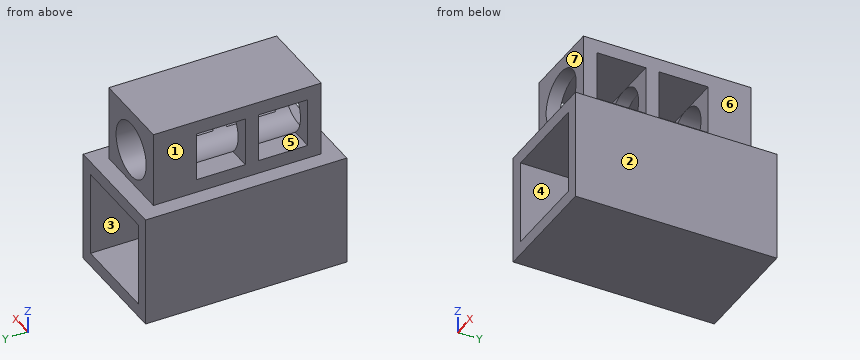
```python
from build123d import *

# Parameters (mm, degrees)
F0_W     = 13.2
F0_H     = 12.6
F1_DEPTH = 15
F0_W_2   = 12.3
F0_H_2   = 11.3
F0_R     = 4.15
F2_DEPTH = 12.5
F3_W     = 7.3
F3_H     = 7.3
F3_W_2   = 7.299999
F4_DEPTH = 25


with BuildPart() as f1:
    # F0 (on Front) → F1 (new body, symmetric)
    with BuildSketch(Plane.XZ):
        Polygon((8.6, -8.3), (8.6, 8.3), (6.15, 8.3), (-6.15, 8.3), (-8.6, 8.3), (-8.6, -8.3), align=None)
        Rectangle(F0_W, F0_H, mode=Mode.SUBTRACT)
    extrude(amount=F1_DEPTH, both=True)

    # F0 (on Front) → F2 (join, symmetric)
    with BuildSketch(Plane.XZ):
        with Locations((0, 13.95)):
            Rectangle(F0_W_2, F0_H_2)
        with Locations((0, 13.45)):
            Circle(F0_R, mode=Mode.SUBTRACT)
    extrude(amount=F2_DEPTH, both=True)

    # F3 (on face) → F4 (cut)
    with BuildSketch(Plane.YZ.offset(6.15)):
        with Locations((-6.85, 13.95)):
            Rectangle(F3_W, F3_H)
        with Locations((2.449999, 13.95)):
            Rectangle(F3_W_2, F3_H)
    extrude(amount=-F4_DEPTH, mode=Mode.SUBTRACT)


solid = f1.part
```
Work out the finished part from the listing and answer in its coordinate system (mm). Face numbers are marked on the shaded views. A direction names the side the tool comes from. Coordinates: 2 decimals unless noted, no trailing zeros. Loops run counter-clockwise (first coordinate to the right, second up) from the corner with the lowest first, then second, coordinate; pieces in that order, holes last. Notation, with made-up numbers: (53.5, -31.75) - (71.5, -31.75) arc R23 cw to (71.5, -17.75) - close; hole circle Ø10 at (54, -14.5). An arc over 180 degrees is marked (long way). Use a Markdown table: item, result.
Item 1: Find section B-B, the plane y = -10. Determine the outline of the cut face in (x, z), and give its area (3 significant figures).
Evaluation:
| item | result |
|---|---|
| outline | (-8.6, -8.3) - (8.6, -8.3) - (8.6, 8.3) - (6.15, 8.3) - (6.15, 10.3) - (2.7, 10.3) arc R4.15 cw to (-2.7, 10.3) - (-6.15, 10.3) - (-6.15, 8.3) - (-8.6, 8.3) - close; (-6.15, 17.6) - (6.15, 17.6) - (6.15, 19.6) - (-6.15, 19.6) - close; hole (-6.6, -6.3) - (6.6, -6.3) - (6.6, 6.3) - (-6.6, 6.3) - close |
| area | 165 mm2 |
Item 2: Given pin 1 Ø12.5 at (y, z) = (-1, 12.5) entering from +X; pin 2 Ø1.8 at (x, z) = (4.5, 14.5) entering from -Y; pin 3 Ø3 at (x, z) = (-3, 12.5) entering from +Y; pin 4 Ø2 at (y, z) = (10, 9.5) entering from +X, each flat-ended and moving along its own axis, determine where each tip first touches the part or whether it passes through.
Evaluation:
| item | result |
|---|---|
| pin 1 | stops at x = 8.6 |
| pin 2 | stops at y = -12.5 |
| pin 3 | stops at y = 12.5 |
| pin 4 | stops at x = 6.15 |
Item 3: The mould has two halves that part along X. Classify the marked faces 1, 2 and 3: +X half, -X half, draft (parallel to the pull), parting line (faces both ways), or undercut.
Evaluation:
| item | result |
|---|---|
| face 1 | -X half |
| face 2 | +X half |
| face 3 | undercut |
Item 4: Find section D-D, the plane y = -2.25. Determine the outline of the cut face in (x, z).
Evaluation:
| item | result |
|---|---|
| outline | (-8.6, -8.3) - (8.6, -8.3) - (8.6, 8.3) - (6.15, 8.3) - (6.15, 19.6) - (-6.15, 19.6) - (-6.15, 8.3) - (-8.6, 8.3) - close; hole (-6.6, -6.3) - (6.6, -6.3) - (6.6, 6.3) - (-6.6, 6.3) - close; hole circle Ø8.3 at (0, 13.45) |
Item 5: Consider probe 1 along Z at (x, y) = (0, -7.25); probe 2 along Z at (x, y) = (4, -7); probe 3 along Y at (x, z) = (4, 16.5). Determine where each line is inside the solid, lowest interval first. Write a range as from..to.
Evaluation:
| item | result |
|---|---|
| probe 1 | z = -8.3..-6.3, 6.3..9.3, 17.6..19.6 |
| probe 2 | z = -8.3..-6.3, 6.3..10.3, 17.6..19.6 |
| probe 3 | y = -12.5..-10.5, -3.2..-1.2, 6.1..12.5 |
Item 6: For the marked faces 4, 5, 6 and 7, determine the directions among +Z, -Z, +X, -X, +Y, -Y from which every point of the face is accessible in a straight line to the end or side of a thin tool.
Evaluation:
| item | result |
|---|---|
| face 4 | +Y, -Y |
| face 5 | +X, -X |
| face 6 | +Z, +X, +Y, -Y |
| face 7 | +Z, +X, -X, -Y |
Item 7: Find section A-A, the plane x = -5.75. Determine the outline of the cut face in (y, z).
Evaluation:
| item | result |
|---|---|
| outline | (-15, -8.3) - (15, -8.3) - (15, -6.3) - (-15, -6.3) - close; (-15, 6.3) - (15, 6.3) - (15, 8.3) - (12.5, 8.3) - (12.5, 19.6) - (-12.5, 19.6) - (-12.5, 8.3) - (-15, 8.3) - close; hole (-10.5, 10.3) - (-3.2, 10.3) - (-3.2, 17.6) - (-10.5, 17.6) - close; hole (-1.2, 10.3) - (6.1, 10.3) - (6.1, 17.6) - (-1.2, 17.6) - close |
Item 8: Find section C-C, the plane z = 2.5. Determine the outline of the cut face in (x, y), and give its area (3 significant figures).
Evaluation:
| item | result |
|---|---|
| outline | (-8.6, -15) - (-6.6, -15) - (-6.6, 15) - (-8.6, 15) - close; (6.6, -15) - (8.6, -15) - (8.6, 15) - (6.6, 15) - close |
| area | 120 mm2 |
